CAD build for the part. Positions are in the model's coordinates, mm. A direction names the side the tool comes from. Coordinates: 2 decimals unless noted, no trailing zeros. Loops run counter-clockwise (first coordinate to the right, second up) from the corner with the lowest first, then second, coordinate; pieces in that order, holes last. Notation, with made-up numbers: (26, -19) -> (54, -19) arc R19 cw to (54, 13) -> close; hole circle Ø9 at (81, -22.5). An arc over 180 degrees is marked (long way). Return JSON: item names as keys, results as strings. Group by question number.
(1) Probe L1, parallel to X at y = -6, z = 10.25; L2, parallel to Y at x = 0, z = 5; L3, parallel to X at y = 4, z = 11.5. List the from-to ranges inside material, lowest first.
(2) Saw through at C-C on z = 8.5. Give the number of separate pieces and of enclosed holes in the cut face, then the cut area to 3 significant figures.
(3) Flat gauge pins, fed straight in: pin 1 Ø5 at (x, z) = (3, 4) entering from +Y; pin 2 Ø8 at (y, z) = (1, 6.5) entering from -X; pin 3 Ø7.5 at (x, y) = (0, 0) entering from +Z; pin 4 Ø4 at (y, z) = (5.5, 8) entering from +X. Where does each tip first touch, or does it go through?
(4) Mould opens along X. For faces 1 (the face through (2, 5, 14.525)), 2 (the face through (-1.03, -4.637, 7.161)), 3 (the face through (0.358, 9.455, 8.086)) say: pulls with the +X half, pulls with the -X half, needs draft (parallel to the pull), parting line crosses it, or undercut.
(5) Saw through at D-D on y = 3.25. Write the cut outline in (x, z) (3 decimals).
(6) Tool access for faces 4 (the face through (0, -8.575, 6)), 5 (the face through (4.8, 8.4, 1.825)): list every direction of +Z, -Z, +X, -X, +Y, -Y with a clear straight run to the whole face (end or side of a thin tool).
```python
from build123d import *

# Parameters (mm, degrees)
SKETCH1_R           = 4.750000025
BOSS_EXTRUDE1_DEPTH = 14.524999906
SKETCH3_R           = 1.474999971
CUT_EXTRUDE1_DEPTH  = 19.05
BOSS_EXTRUDE2_DEPTH = 1.825


with BuildPart() as part:
    # Sketch1 → Boss-Extrude1 (new body)
    with BuildSketch(Plane.XY):
        with BuildLine():
            Line((-3.998602683, -8.575031127), (3.998602683, -8.575031127))
            ThreePointArc((3.998602683, -8.575031127), (0, 9.4615), (-3.998602683, -8.575031127))
        make_face()
        Circle(SKETCH1_R, mode=Mode.SUBTRACT)
    extrude(amount=BOSS_EXTRUDE1_DEPTH)

    # Sketch3 → Cut-Extrude1 (cut)
    with BuildSketch(Plane(origin=(0, 0, 0), x_dir=(-1, 0, 0), z_dir=(0, 0, -1))):
        with Locations((5.126524148, -5.126524148)):
            Circle(SKETCH3_R)
        with Locations((-5.126524148, -5.126524148)):
            Circle(SKETCH3_R)
        with Locations((-5.126524148, 5.126524148)):
            Circle(SKETCH3_R)
        with Locations((5.126524148, 5.126524148)):
            Circle(SKETCH3_R)
    extrude(amount=-CUT_EXTRUDE1_DEPTH, mode=Mode.SUBTRACT)

    # Sketch4 → Boss-Extrude2 (add)
    with BuildSketch(Plane.XY):
        with BuildLine():
            Line((-3.998602683, -8.575031127), (-9.367968892, -8.575031127))
            ThreePointArc((-9.367968892, -8.575031127), (0, 12.7), (9.367968892, -8.575031127))
            Line((9.367968892, -8.575031127), (3.998602683, -8.575031127))
            ThreePointArc((3.998602683, -8.575031127), (0, 9.4615), (-3.998602683, -8.575031127))
        make_face()
    extrude(amount=BOSS_EXTRUDE2_DEPTH)


solid = part.part
```
Geometry results:
{
 "1": {"L1": "-7.32 to -6.32, -3.94 to 3.94, 6.32 to 7.32", "L2": "-8.58 to -4.75, 4.75 to 9.46", "L3": "-8.57 to -6.08, -4.17 to -2.56, 2.56 to 4.17, 6.08 to 8.57"},
 "2": {"separate pieces": "1", "enclosed holes": "5", "area": "178 mm²"},
 "3": {"pin 1": "y = 12.58", "pin 2": "x = -9.46", "pin 3": "through", "pin 4": "x = 8.79"},
 "4": {"face 1": "needs draft", "face 2": "undercut", "face 3": "parting line crosses it"},
 "5": {"outline": "(-12.277, 0) -> (-3.464, 0) -> (-3.464, 14.525) -> (-8.886, 14.525) -> (-8.886, 1.825) -> (-12.277, 1.825) -> close; (3.464, 0) -> (12.277, 0) -> (12.277, 1.825) -> (8.886, 1.825) -> (8.886, 14.525) -> (3.464, 14.525) -> close"},
 "6": {"face 4": "+Z, -Z, +X, -X, -Y", "face 5": "+Z"}
}
